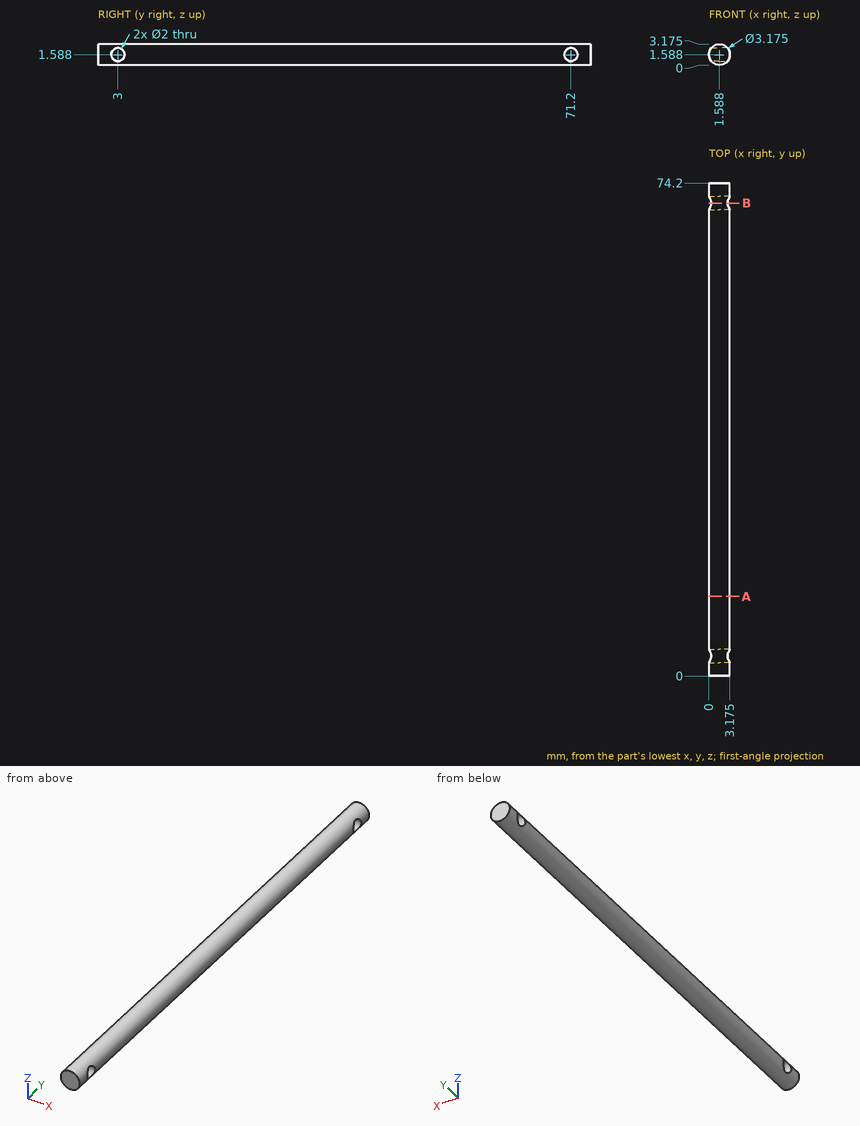
Here's the drawing with two shaded views (mm, measured from the low corner). I have some questions. Round coordinates to 2 decimals unless told otherwise and drop trailing zeros. Loops run counter-clockwise (first coordinate to the right, second up) from the corner with the lowest first, then second, coordinate; pieces in that order, holes last.
1. Suppose I cut it at A-A, the plane y = 12. Please give me the cut outline in (x, z) (1 decimal).
Answers:
outline: circle Ø3.2 at (1.6, 1.6)
2. Will these pins go through, and if not, where does the flat tip stop? pin 1 (1.5 mm diameter, centred on y = 14, z = 2.5, fed in from -X); pin 2 (1 mm diameter, centred on y = 11, z = 2.5, fed in from +X).
Answers:
pin 1: stops at x = 0.01
pin 2: stops at x = 3.12
3. If I drill on probe 1 along Y at (x, z) = (2.2, 1.5) (1 decimal); probe 2 along Y at (x, z) = (0.35, 0.9) (1 decimal); probe 3 along Z at (x, y) = (1.45, 46) (1 decimal), over which ranges is the centre line in solid material (lowest first)?
Answers:
probe 1: y = 0 to 2, 4 to 70.2, 72.2 to 74.2
probe 2: y = 0 to 2.3, 3.7 to 70.5, 71.9 to 74.2
probe 3: z = 0 to 3.2
4. Suppose I cut it at B-B, the plane y = 71.2. Please give me the cut outline in (x, z) (1 decimal).
Answers:
outline: (0.4, 0.6) arc R1.6 ccw to (2.8, 0.6) - close; (0.4, 2.6) - (2.8, 2.6) arc R1.6 ccw to start
